Read the model definition and answer for the solid it produces. Units are mm, in the model's axes. Face numbers are marked on the shaded views. A direction names the side the tool comes from. Coordinates: 2 decimals unless noted, no trailing zeros. Write each loop counter-clockwise with the first axis right and the second up, starting at its lowest first coordinate (ties: lowest second). Pieces come first, ordered by that corner, then holes.
(1) The part is cut by section A-A, the plane x = 11. Determine the outline of the cut face in (y, z).
(2) Which of the six approach directions +Z, -Z, +X, -X, +Y, -Y give full straight-line access (tool end or side, diameter ignored) to the marked faces 5, 6, 7, 8 and 9?
(3) Straight lines are drawn through the part: line 1 along X through (y, z) = (20.75, 8); line 2 along X through (y, z) = (7, 15.5); line 3 along Y through (x, z) = (5.5, 20). For each, find the intervals that lie inside material, in ascending order.
(4) Given pin 1 (4 mm diameter, centred on x = 14.5, y = 17.5, fed in from -Z); pin 2 (12 mm diameter, centred on y = 18, z = 23, fed in from +X); pin 3 (11 mm diameter, centred on y = 12, z = 10.5, fed in from -X); pin 4 (1.2 mm diameter, centred on x = 10.5, y = 13, fed in from +Z), each flat-ended and moving along its own axis, determine where each tip first touches the part or whether it passes through.
(5) Determine the mould class of the marked faces 1, 2, 3 and 4 for opening direction X: pulls with the +X half, pulls with the -X half, needs draft (parallel to the pull), parting line crosses it, or undercut.
(6) The part is cut by section C-C, the plane z = 17.5. Determine the outline of the cut face in (x, y).
(7) The part is cut by section B-B, the plane y = 12. Determine the outline of the cut face in (x, z), and give its area (3 significant figures).
(8) The part is cut by section D-D, the plane x = 40.5. Determine the outline of the cut face in (y, z).
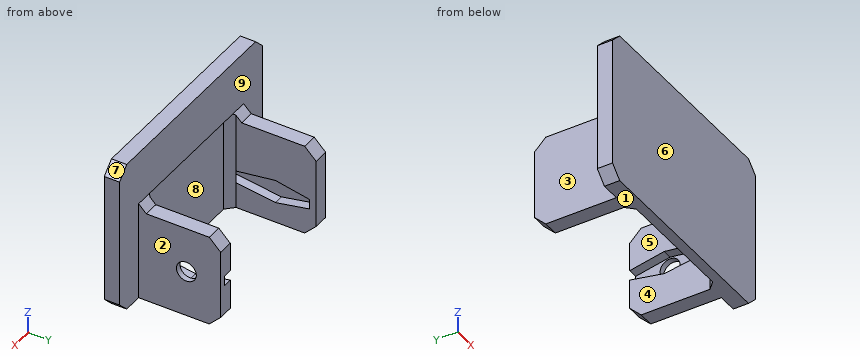
```python
from build123d import *

# Parameters (mm, degrees)
SKETCH1_W           = 60
SKETCH1_H           = 40
BOSS_EXTRUDE1_DEPTH = 4
CHAMFER1_SIZE       = 3
SKETCH2_W           = 36
SKETCH2_H           = 24
CUT_EXTRUDE1_DEPTH  = 1.5
SKETCH3_W           = 4
SKETCH3_H           = 24
BOSS_EXTRUDE2_DEPTH = 23
CHAMFER2_SIZE       = 3
CHAMFER3_SIZE       = 2
CHAMFER4_SIZE       = 2
CHAMFER5_SIZE       = 2
CUT_EXTRUDE2_DEPTH  = 2.5
SKETCH7_R           = 2.604037506
CUT_EXTRUDE3_DEPTH  = 70.285640648
CUT_EXTRUDE4_DEPTH  = 2.5


with BuildPart() as part:
    # Sketch1 → Boss-Extrude1 (new body)
    with BuildSketch(Plane(origin=(0, 0, 0), x_dir=(1, 0, 0), z_dir=(0, 1, 0))):
        with Locations((30, -20)):
            Rectangle(SKETCH1_W, SKETCH1_H)
    extrude(amount=BOSS_EXTRUDE1_DEPTH)

    # Chamfer1
    chamfer1_edges = [part.edges().sort_by_distance(p)[0] for p in [
        (0, 2, 0),
        (60, 2, 0),
        (60, 2, 40),
        (0, 2, 40),
    ]]
    chamfer(chamfer1_edges, length=CHAMFER1_SIZE)

    # Sketch2 → Cut-Extrude1 (cut)
    with BuildSketch(Plane(origin=(0, 4, 0), x_dir=(1, 0, 0), z_dir=(0, 1, 0))):
        with Locations((30, -12)):
            Rectangle(SKETCH2_W, SKETCH2_H)
    extrude(amount=-CUT_EXTRUDE1_DEPTH, mode=Mode.SUBTRACT)

    # Sketch3 → Boss-Extrude2 (add)
    with BuildSketch(Plane(origin=(0, 2.5, 0), x_dir=(1, 0, 0), z_dir=(0, 1, 0))):
        with Locations((50, -12)):
            Rectangle(SKETCH3_W, SKETCH3_H)
        with Locations((10, -12)):
            Rectangle(SKETCH3_W, SKETCH3_H)
    extrude(amount=BOSS_EXTRUDE2_DEPTH)

    # Chamfer2
    chamfer2_edges = [part.edges().sort_by_distance(p)[0] for p in [
        (50, 25.5, 24),
        (50, 25.5, 0),
        (10, 25.5, 0),
        (10, 25.5, 24),
    ]]
    chamfer(chamfer2_edges, length=CHAMFER2_SIZE)

    # Chamfer3
    chamfer3_edges = [part.edges().sort_by_distance(p)[0] for p in [
        (50, 4, 24),
        (10, 4, 24),
    ]]
    chamfer(chamfer3_edges, length=CHAMFER3_SIZE)

    # Chamfer4
    # the kernel refuses this chamfer: 2 mm, written as the material it takes off along each edge
    with BuildSketch(Plane(origin=(48, 4, 24), x_dir=(0, -0.9996219169112968, -0.027495876610585623), z_dir=(-1, 0, 0))) as chamfer4_piece_1_section:
        Polygon((CHAMFER4_SIZE * 0.999621916911, CHAMFER4_SIZE * 0.0274958766106), (-CHAMFER4_SIZE * 0.0274958766106, CHAMFER4_SIZE * 0.999621916911), (0, 0), align=None)
    chamfer4_piece_1 = extrude(amount=36, mode=Mode.PRIVATE)
    chamfer4_piece_1 = split(chamfer4_piece_1, bisect_by=Plane(origin=(30, 2.5, 24.699033576), z_dir=(0, 1, 0)), keep=Keep.TOP, mode=Mode.PRIVATE)
    chamfer4_piece_1 = split(chamfer4_piece_1, bisect_by=Plane(origin=(30, 4.361799404, 25.638200596), z_dir=(0, -0.7071067811865476, -0.7071067811865476)), keep=Keep.TOP, mode=Mode.PRIVATE)
    add(chamfer4_piece_1, mode=Mode.SUBTRACT)

    # Chamfer5
    # the kernel refuses this chamfer: 2 mm, written as the material it adds along each edge
    with BuildSketch(Plane(origin=(12, 2.5, 29.643365976), x_dir=(-0.027495876610586487, 0.9996219169112968, 0), z_dir=(0, 0, -1))) as chamfer5_piece_1_section:
        Polygon((CHAMFER5_SIZE * 0.999621916911, CHAMFER5_SIZE * 0.0274958766106), (-CHAMFER5_SIZE * 0.0274958766106, CHAMFER5_SIZE * 0.999621916911), (0, 0), align=None)
    chamfer5_piece_1 = extrude(amount=29.643365976, mode=Mode.PRIVATE)
    chamfer5_piece_1 = split(chamfer5_piece_1, bisect_by=Plane(origin=(12.696713147, 10.276643426, 19.723356574), z_dir=(0, -0.7071067811865476, -0.7071067811865476)), keep=Keep.TOP, mode=Mode.PRIVATE)
    add(chamfer5_piece_1)
    with BuildSketch(Plane(origin=(48, 2.5, 29.643365976), x_dir=(-0.9996219169112968, -0.027495876610586296, 0), z_dir=(0, 0, -1))) as chamfer5_piece_2_section:
        Polygon((CHAMFER5_SIZE * 0.999621916911, CHAMFER5_SIZE * 0.0274958766106), (-CHAMFER5_SIZE * 0.0274958766106, CHAMFER5_SIZE * 0.999621916911), (0, 0), align=None)
    chamfer5_piece_2 = extrude(amount=29.643365976, mode=Mode.PRIVATE)
    chamfer5_piece_2 = split(chamfer5_piece_2, bisect_by=Plane(origin=(47.833064516, 10.624596774, 19.375403226), z_dir=(0, -0.7071067811865476, -0.7071067811865476)), keep=Keep.TOP, mode=Mode.PRIVATE)
    add(chamfer5_piece_2)

    # Sketch4 → Cut-Extrude2 (cut)
    with BuildSketch(Plane.ZY.offset(-48)):
        Polygon((9.05620064, 16.5), (10.815025537, 25.5), (13.420692052, 25.5), (15.179516949, 16.5), (13.420692052, 4), (10.815025537, 4), align=None)
    extrude(amount=-CUT_EXTRUDE2_DEPTH, mode=Mode.SUBTRACT)

    # Sketch7 → Cut-Extrude3 (cut, through all)
    with BuildSketch(Plane.ZY.offset(-50.5)):
        with Locations((12.117858795, 16.5)):
            Circle(SKETCH7_R)
    extrude(amount=-CUT_EXTRUDE3_DEPTH, mode=Mode.SUBTRACT)

    # Sketch8 → Cut-Extrude4 (cut)
    with BuildSketch(Plane(origin=(12, 0, 0), x_dir=(0, 0, -1), z_dir=(1, 0, 0))):
        Polygon((-11.53257408, 14.821897089), (-9.773749183, 23.821897089), (-7.168082669, 23.821897089), (-5.409257772, 14.821897089), (-7.168082669, 2.321897089), (-9.773749183, 2.321897089), align=None)
    extrude(amount=-CUT_EXTRUDE4_DEPTH, mode=Mode.SUBTRACT)


solid = part.part
```
Computed:
1. outline: (0, 0) - (22.5, 0) - (25.5, 3) - (25.5, 21) - (22.5, 24) - (6, 24) - (4, 26) - (4, 40) - (0, 40) - close; hole (2.32, 7.17) - (14.82, 5.41) - (23.82, 7.17) - (23.82, 9.77) - (14.82, 11.53) - (2.32, 9.77) - close
2. face 5: +Z, -Z, +Y
2. face 6: +Z, -Z, +X, -X, -Y
2. face 7: +Z, +X, +Y, -Y
2. face 8: -Z, +Y
2. face 9: +Z, +Y
3. line 1: x = 8 to 9.5, 48 to 52
3. line 2: x = 8 to 12, 48 to 52
3. line 3: y = 0 to 4
4. pin 1: passes through
4. pin 2: stops at x = 52
4. pin 3: stops at x = 8
4. pin 4: stops at z = 24
5. face 1: needs draft
5. face 2: pulls with the +X half
5. face 3: pulls with the -X half
5. face 4: undercut
6. outline: (0, 0) - (60, 0) - (60, 4) - (52, 4) - (52, 25.5) - (48, 25.5) - (48, 4.5) - (46, 2.5) - (14, 2.5) - (12, 4.5) - (12, 25.5) - (8, 25.5) - (8, 4) - (0, 4) - close
7. outline: (8, 0) - (12, 0) - (12, 5.81) - (9.5, 5.81) - (9.5, 11.14) - (12, 11.14) - (12, 24) - (8, 24) - close; (48, 0) - (52, 0) - (52, 24) - (48, 24) - (48, 14.55) - (50.5, 14.55) - (50.5, 9.69) - (48, 9.69) - close
7. area: 167 mm2
8. outline: (0, 0) - (2.5, 0) - (2.5, 24.5) - (4, 26) - (4, 40) - (0, 40) - close
